Geometry check sheet. Reference: drawing and pictorial views, mm from the part's lowest x, y, z. A direction names the side the tool comes from. Round coordinates to 2 decimals unless told otherwise and drop trailing zeros. Loops run counter-clockwise (first coordinate to the right, second up) from the corner with the lowest first, then second, coordinate; pieces in that order, holes last. Notation, with made-up numbers: (29, 71) -> (61, 71) arc R18 ccw to (61, 79) -> close; hole circle Ø5 at (6.5, 30.5). An arc over 180 degrees is marked (long way). Use one line per item in the form item = value. Start each with the question number.
(1) Material ranges on probe 1 along Z at (x, y) = (1.5, 3.4); probe 2 along Y at (x, z) = (11.5, 16); probe 3 along Y at (x, z) = (2, 10.5), recorded low to high. Write a range as [from, to].
(2) Set-up check for the marked faces 5, 6 and 7: record each of +Z, -Z, +X, -X, +Y, -Y from which the full face is reachable in a straight line by a thin tool's end or side.
(3) Sectioned sample at C-C (z = 18.25). Record the cut outline in (x, y).
(4) Sectioned sample at D-D (x = 5.25). Record the cut outline in (y, z).
(5) Go/stop test with flat-tipped pins: pin 1 (0.5 mm diameter, centred on x = 8, y = 4, fed in from -Z); pin 2 (0.5 mm diameter, centred on x = 1, z = 13.5, fed in from +Y); pin 3 (0.9 mm diameter, centred on x = 13, z = 9.5, fed in from +Y). Record where each tip stops, or that it passes through.
(6) Draft check along X on the marked faces 1, 2, 3 and 4. Enter one of: released by +X, released by -X, zero draft, split by the parting line, or undercut.
(7) Sectioned sample at A-A (z = 7.75). Record the cut outline in (x, y).
(8) Sectioned sample at B-B (y = 2.2). Record the cut outline in (x, z), and give its area (3 significant figures).
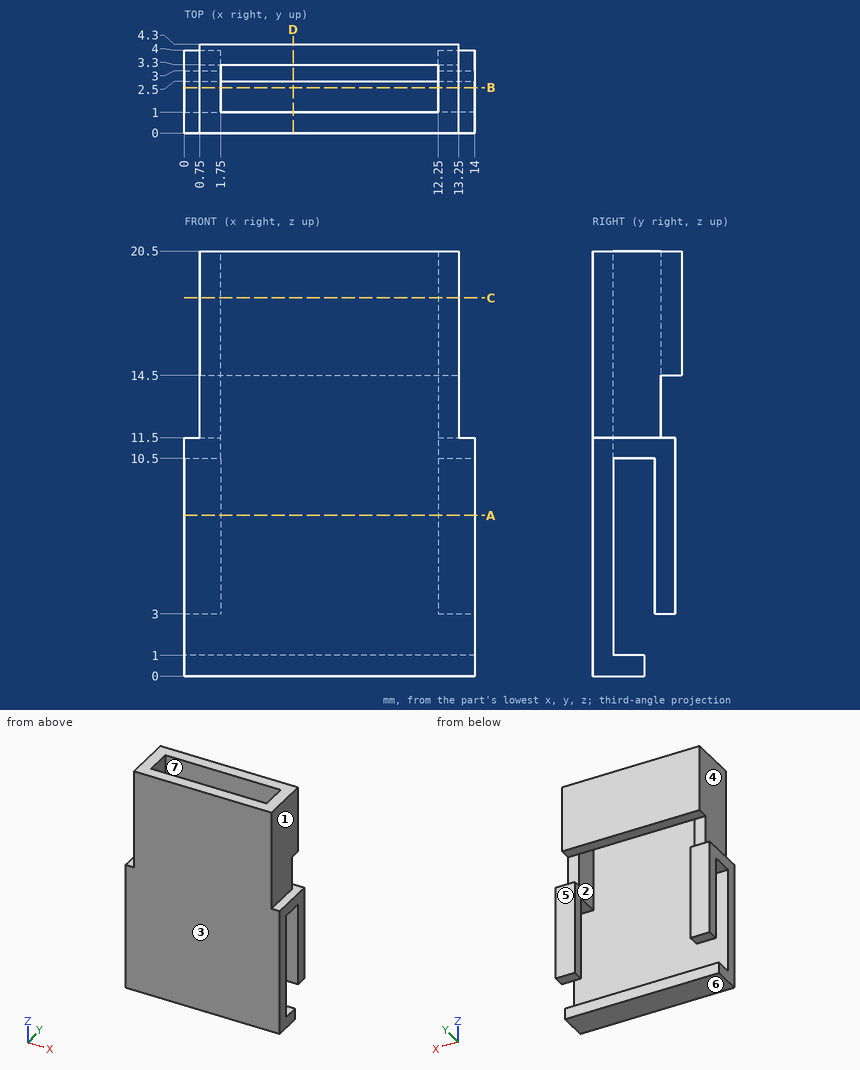
Checks:
q1.probe_1 = [3, 11.5], [14.5, 20.5]
q1.probe_2 = [0, 1], [3.3, 4.3]
q1.probe_3 = [0, 1]
q2.face_5 = -Z, +X, -X, +Y
q2.face_6 = -Z, +X, -X, +Y, -Y
q2.face_7 = +Z, -Z
q3.outline = (0.75, 0) -> (13.25, 0) -> (13.25, 4.3) -> (0.75, 4.3) -> close; hole (1.75, 1) -> (12.25, 1) -> (12.25, 3.3) -> (1.75, 3.3) -> close
q4.outline = (0, 0) -> (2.5, 0) -> (2.5, 1) -> (1, 1) -> (1, 20.5) -> (0, 20.5) -> close; (3.3, 14.5) -> (4.3, 14.5) -> (4.3, 20.5) -> (3.3, 20.5) -> close
q5.pin_1 = 14.5
q5.pin_2 = 3.3
q5.pin_3 = 4
q6.face_1 = released by +X
q6.face_2 = undercut
q6.face_3 = zero draft
q6.face_4 = released by -X
q7.outline = (0, 0) -> (14, 0) -> (14, 1) -> (0, 1) -> close; (0, 3) -> (1.75, 3) -> (1.75, 4) -> (0, 4) -> close; (12.25, 3) -> (14, 3) -> (14, 4) -> (12.25, 4) -> close
q8.outline = (0, 0) -> (14, 0) -> (14, 1) -> (0, 1) -> close; (0, 10.5) -> (1.75, 10.5) -> (1.75, 20.5) -> (0.75, 20.5) -> (0.75, 11.5) -> (0, 11.5) -> close; (12.25, 10.5) -> (14, 10.5) -> (14, 11.5) -> (13.25, 11.5) -> (13.25, 20.5) -> (12.25, 20.5) -> close
q8.area = 35.5 mm2
